The model under review builds one solid part; all positions refer to its coordinate system, in mm. Round coordinates to 2 decimals unless told otherwise and drop trailing zeros. Order: outer loops, then holes, each group sorted by start corner. A loop starts at its lowest first (then second) coordinate and runs counter-clockwise, first axis right, second up.
1) Consider section A-A (x = -62.25). Give the boundary of the cut face in (y, z).
2) Clearance check with a flat-ended pin moving along its axis: P1, Ø4, axis at x = -62.25, z = 62.25, coming from the -Y side. State where the tip first meets the part, or that it passes through.
3) To check wall thickness, follow L1, parallel to X at y = 6, z = 62.25. State the ranges of the line that lie inside material, in increasing order.
4) Consider section B-B (z = 62.25). Give the boundary of the cut face in (x, y), then the cut area to 3 significant figures.
5) Mouldability with a two-part tool opening along Z and no side actions: class faces 1 (the face through (-64.282, 12.152, -61.407)), 2 (the face through (69, 12, 68)), 3 (the face through (-70, 12, 1)), 4 (the face through (-69, 12, -68)) as pulls with the +Z half, pulls with the -Z half, needs draft (parallel to the pull), parting line crosses it, or undercut.
Autodesk Inventor part; units mm, degrees
ref_plane "YZ Plane" through (0, 0, 0) normal (1, 0, 0) x (0, 1, 0)
ref_plane "XZ Plane" through (0, 0, 0) normal (0, 1, 0) x (-1, 0, 0)
ref_plane "XY Plane" through (0, 0, 0) normal (0, 0, 1) x (1, 0, 0)
sketch "Sketch1" plane through (0, 0, 0) normal (0, 1, 0) x (-1, 0, 0)
  line L0 (-65, 70) -> (65, 70)
  line L1 (70, 65) -> (70, -65)
  line L2 (65, -70) -> (-65, -70)
  line L3 (-70, -65) -> (-70, 65)
  line L4 (-70, 70) -> (70, -70) construction
  line L5 (70, 70) -> (-70, -70) construction
  arc A0 (70, 65) -> (65, 70) centre (65, 65) ccw
  arc A1 (-65, 70) -> (-70, 65) centre (-65, 65) ccw
  arc A2 (-70, -65) -> (-65, -70) centre (-65, -65) ccw
  arc A3 (65, -70) -> (70, -65) centre (65, -65) ccw
  line L6 (0, 70) -> (0, 62.25)
  line L7 (70, 0) -> (62.25, 0)
  line L8 (0, -70) -> (0, -62.25)
  line L9 (-70, 0) -> (-62.25, 0)
  line L10 (-62.25, 62.25) -> (-62.25, -62.25)
  line L11 (-62.25, -62.25) -> (62.25, -62.25)
  line L12 (62.25, -62.25) -> (62.25, 62.25)
  line L13 (62.25, 62.25) -> (-62.25, 62.25)
  line L14 (-62.25, 62.25) -> (62.25, -62.25) construction
  line L15 (-62.25, -62.25) -> (62.25, 62.25) construction
  circle A4 centre (62.25, -62.25) radius 2.2
  circle A5 centre (-62.25, -62.25) radius 2.2
  circle A6 centre (-62.25, 62.25) radius 2.2
  circle A7 centre (62.25, 62.25) radius 2.2
  arc A8 (60.05, 62.25) -> (62.25, 60.05) centre (62.25, 62.25) ccw
  arc A9 (62.25, -60.05) -> (60.05, -62.25) centre (62.25, -62.25) ccw
  arc A10 (-60.05, -62.25) -> (-62.25, -60.05) centre (-62.25, -62.25) ccw
  arc A11 (-62.25, 60.05) -> (-60.05, 62.25) centre (-62.25, 62.25) ccw
  arc A12 (-60.05, -62.25) -> (-62.25, -60.05) centre (-62.25, -62.25) ccw
  point P0 (0, 0)
  dimension "d0" = 140
  dimension "d1" = 140
  dimension "d2" = 5
  dimension "d3" = 7.75
  dimension "d4" = 7.75
  dimension "d5" = 7.75
  dimension "d6" = 7.75
  dimension "d7" = 4.4
  dimension "d8" = 4.4
  dimension "d9" = 4.4
  dimension "d10" = 4.4
extrude "Extrusion1" add sketch "Sketch1" along normal blind 24.65 contours L0 L6 L13 A6 L10 L9 L3 A1 | L0 A0 L1 L7 L12 A7 L13 L6 | L13 A7 L12 A4 L11 A5 L10 A6 | L9 L10 A5 L11 L8 L2 A2 L3 | L1 A3 L2 L8 L11 A4 L12 L7 | A5 L11 L10 | L10 L11 A5
sketch "Sketch2" plane through (0, 24.65, 0) normal (0, 1, 0) x (1, 0, 0)
  circle A0 centre (62.25, -62.25) radius 2.2
  line L0 (62.25, -62.25) -> (62.25, 62.25)
  line L1 (65, 70) -> (-65, 70)
  circle A1 centre (-62.25, 62.25) radius 2.2
  line L2 (-62.25, 62.25) -> (62.25, 62.25)
  circle A2 centre (62.25, 62.25) radius 2.2
  point P0 (0, 0)
  dimension "d13" = 4.4
extrude "Extrusion2" cut sketch "Sketch2" against normal up to next contours A2 L2 L0 | L0 L2 A2
properties part number "BaseFan"
Answer below:
1. outline: (0, -70) - (24.65, -70) - (24.65, -64.45) - (0, -64.45) - close; (0, -60.05) - (24.65, -60.05) - (24.65, 60.05) - (0, 60.05) - close; (0, 64.45) - (24.65, 64.45) - (24.65, 70) - (0, 70) - close
2. P1: passes through
3. L1: x = -70 to -64.45, -60.05 to 60.05, 64.45 to 70
4. outline: (-70, 0) - (-64.45, 0) - (-64.45, 24.65) - (-70, 24.65) - close; (-60.05, 0) - (60.05, 0) - (60.05, 24.65) - (-60.05, 24.65) - close; (64.45, 0) - (70, 0) - (70, 24.65) - (64.45, 24.65) - close
4. area: 3,230 mm2
5. face 1: undercut
5. face 2: pulls with the +Z half
5. face 3: needs draft
5. face 4: pulls with the -Z half
